Design review of the part built by this model. Coordinates are the model's own, in mm. A direction names the side the tool comes from. Give positions to 0.01 mm unless a question says otherwise; leave off trailing zeros. Loops run counter-clockwise (first coordinate to the right, second up) from the corner with the lowest first, then second, coordinate; pieces in that order, holes last. Notation, with made-up numbers: M 75.25,24.5 L 100.25,24.5 A21 ccw 100.25,30.5 Z; hole C -22.5,-14.75 d11. An arc over 180 degrees is marked long. Use a Markdown table: item, result. Add a question column.
(1) Draft analysis for pull direction Y (two halves, no side actions). For faces 4 (the face through (-13, -8.2, 2)), 5 (the face through (-13.774, -2.092, 1.633)), 6 (the face through (9, 0, 0)), state which applies: pulls with the +Y half, pulls with the -Y half, needs draft (parallel to the pull), parting line crosses it, or undercut.
(2) Add section D-D, the plane y = -5.25. Give the boundary of the cut face in (x, z).
(3) Add section B-B, the plane z = 1.25. Give the boundary of the cut face in (x, y) (3 decimals), then the cut area to 3 significant figures.
(4) For probe 1 along X at (y, z) = (1, 3.45); probe 2 along X at (y, z) = (-5.25, 1.15); probe 3 along Z at (x, y) = (4, -0.25), list the stretches that pass through material, from the lowest coordinate up.
(5) Add section A-A, the plane x = 21.5. Give the boundary of the cut face in (y, z).
(6) Insertion check: pin 1 Ø1.5 at (x, z) = (10, 0.5) entering from -Y; pin 2 Ø2 at (x, z) = (7, 1) entering from +Y; pin 3 Ø5.5 at (x, y) = (4, 0) entering from -Z. Each pin has a flat end and moves straight along its axis. Give the tip position at first contact, or say it passes through.
(7) For faces 1 (the face through (0, 1.5, 1)), 2 (the face through (-14, -3.2, 3)), 3 (the face through (-15.194, -0.021, 1.233)), list the 3-axis set-ups (+Z, -Z, +X, -X, +Y, -Y) from which the entire face can be reached by the end or side of a thin tool; tool diameter is ignored.
(8) Add section C-C, the plane x = -12.85. Give the boundary of the cut face in (y, z).
```python
from build123d import *

# Parameters (mm, degrees)
SCHIZZO1_W                   = 33
SCHIZZO1_H                   = 3
ESTRUSIONE_ESTRUSIONE1_DEPTH = 2.5
TAGLIO_ESTRUSIONE1_DEPTH     = 17.955824958
SCHIZZO3_R                   = 1
ESTRUSIONE_ESTRUSIONE2_DEPTH = 1.7
SCHIZZO5_R                   = 2.5
ESTRUSIONE_ESTRUSIONE3_DEPTH = 5
SMUSSO2_SIZE                 = 0.5
SCHIZZO8_W                   = 4
SCHIZZO8_H                   = 5
ESTRUSIONE_ESTRUSIONE6_DEPTH = 10
TAGLIO_ESTRUSIONE3_DEPTH     = 29.232118234
TAGLIO_ESTRUSIONE4_START     = -5
TAGLIO_ESTRUSIONE4_DEPTH     = 5


with BuildPart() as part:
    # Schizzo1 → Estrusione-Estrusione1 (new body)
    with BuildSketch(Plane.XY):
        Rectangle(SCHIZZO1_W, SCHIZZO1_H)
    extrude(amount=ESTRUSIONE_ESTRUSIONE1_DEPTH)

    # Schizzo2 → Taglio-Estrusione1 (cut, through all)
    with BuildSketch(Plane.XZ.offset(1.5)):
        Polygon((-16.5, 0), (-13.85, 2.5), (-16.5, 2.5), align=None)
    extrude(amount=-TAGLIO_ESTRUSIONE1_DEPTH, mode=Mode.SUBTRACT)

    # Schizzo3 → Estrusione-Estrusione2 (add)
    with BuildSketch(Plane.XZ.offset(1.5)):
        with Locations(Location((-12.85, 1.25, 0), (0, 0, 180))):
            Circle(SCHIZZO3_R)
    extrude(amount=ESTRUSIONE_ESTRUSIONE2_DEPTH)

    # Schizzo5 → Estrusione-Estrusione3 (add)
    with BuildSketch(Plane.XZ.offset(3.2)):
        with Locations((-12.85, 1.25)):
            Circle(SCHIZZO5_R)
    extrude(amount=ESTRUSIONE_ESTRUSIONE3_DEPTH)

    # Smusso2
    smusso2_edges = [part.edges().sort_by_distance(p)[0] for p in [
        (-11.85, -3.2, 1.25),
    ]]
    chamfer(smusso2_edges, length=SMUSSO2_SIZE)

    # Schizzo8 → Estrusione-Estrusione6 (add)
    with BuildSketch(Plane(origin=(16.5, 0, 0), x_dir=(0, 0, -1), z_dir=(1, 0, 0))):
        with Locations((-2, 1)):
            Rectangle(SCHIZZO8_W, SCHIZZO8_H)
    extrude(amount=ESTRUSIONE_ESTRUSIONE6_DEPTH)

    # Schizzo9 → Taglio-Estrusione3 (cut, through all)
    with BuildSketch(Plane.XY.offset(4)):
        with BuildLine():
            ThreePointArc((22.75, 1), (21.787191151, 2.216561237), (20.381966011, 1.559016994))
            Line((20.381966011, 1.559016994), (22.618033989, 0.440983006))
            ThreePointArc((22.618033989, 0.440983006), (22.716561237, 0.712808849), (22.75, 1))
        make_face()
        with BuildLine():
            Line((22.618033989, 0.440983006), (20.381966011, 1.559016994))
            ThreePointArc((20.381966011, 1.559016994), (20.940983006, -0.118033989), (22.618033989, 0.440983006))
        make_face()
    extrude(amount=-TAGLIO_ESTRUSIONE3_DEPTH, mode=Mode.SUBTRACT)

    # Schizzo10 → Taglio-Estrusione4 (cut)
    with BuildSketch(Plane.XZ.offset(8.2).offset(TAGLIO_ESTRUSIONE4_START)):
        with BuildLine():
            Line((-11.35, -0.75), (-14.35, -0.75))
            ThreePointArc((-14.35, -0.75), (-12.85, -1.25), (-11.35, -0.75))
        make_face()
    extrude(amount=TAGLIO_ESTRUSIONE4_DEPTH, mode=Mode.SUBTRACT)


solid = part.part
```
Established:
| question | item | result |
|---|---|---|
| 1 | face 4 | pulls with the -Y half |
| 1 | face 5 | undercut |
| 1 | face 6 | needs draft |
| 2 | outline | M -14.35,-0.75 L -11.35,-0.75 A2.5 ccw long Z |
| 3 | outline | M -15.35,-8.2 L -10.35,-8.2 L -10.35,-3.2 L -11.35,-3.2 L -11.85,-2.7 L -11.85,-1.5 L 26.5,-1.5 L 26.5,3.5 L 16.5,3.5 L 16.5,1.5 L -15.175,1.5 L -15.175,-1.5 L -13.85,-1.5 L -13.85,-2.7 L -14.35,-3.2 L -15.35,-3.2 Z; hole C 21.5,1 d2.5 |
| 3 | area | 169 mm^2 |
| 4 | probe 1 | 16.5 to 20.25, 22.75 to 26.5 |
| 4 | probe 2 | -15.35 to -10.35 |
| 4 | probe 3 | 0 to 2.5 |
| 5 | outline | M -1.5,0 L -0.25,0 L -0.25,4 L -1.5,4 Z; M 2.25,0 L 3.5,0 L 3.5,4 L 2.25,4 Z |
| 6 | pin 1 | y = -1.5 |
| 6 | pin 2 | y = 1.5 |
| 6 | pin 3 | z = 0 |
| 7 | face 1 | +Z, -Z, -X, +Y |
| 7 | face 2 | none |
| 7 | face 3 | +Z, -X, +Y |
| 8 | outline | M -8.2,-0.75 L -3.2,-0.75 L -3.2,-0.25 L -2.7,0.25 L -1.5,0.25 L -1.5,0 L 1.5,0 L 1.5,2.5 L -1.5,2.5 L -1.5,2.25 L -2.7,2.25 L -3.2,2.75 L -3.2,3.75 L -8.2,3.75 Z |
